Read the model definition and answer for the solid it produces. Units are mm, in the model's axes. A direction names the side the tool comes from. Coordinates: 2 decimals unless noted, no trailing zeros. Loops run counter-clockwise (first coordinate to the right, second up) from the corner with the lowest first, then second, coordinate; pieces in that order, holes last. Notation, with made-up numbers: (35, 85) -> (58, 85) arc R24 ccw to (58, 111) -> close; hole circle Ø5 at (67, 36). An arc over 180 degrees is marked (long way). Answer as a JSON object with one key per item and string values. Group by question number.
1) Determine the mould class of faces 1 (the face through (-17, 4, -63.5)), 2 (the face through (17, -1, -69.85)), 3 (the face through (-17, 4, 63.5)), 4 (the face through (1219.2, -40, 0)) for opening direction Z: released by +Z, released by -Z, zero draft, split by the parting line, or undercut.
2) Flat-ended cylindrical pins translate along their axes: P1, Ø1, axis at x = 168, z = -16.5, coming from the +Y side; P2, Ø15, axis at x = 291.29, z = 11.6, coming from the +Y side. Find the tip coordinate at first contact, or state that the pin passes through.
3) Section A-A, the plane y = -23 is taken. Give the vertices of the cut face in (x, z).
4) Consider probe 1 along Z at (x, y) = (596.5, 34); probe 2 along Y at (x, z) = (801, -51). Determine where each line is inside the solid, lowest interval first. Write a range as [from, to].
5) Section B-B, the plane x = 645 is taken. Give the vertices of the cut face in (y, z), plus the area to 3 significant figures.
6) Which of the six approach directions +Z, -Z, +X, -X, +Y, -Y give full straight-line access (tool end or side, diameter ignored) to faces 5 (the face through (-17, -38.1, -1)), 6 (the face through (17, -44.45, -1))?
from build123d import *

# Parameters (mm, degrees)
F0_W     = 88.9
F0_H     = 139.7
F1_DEPTH = 1219.2
F2_W     = 82.55
F2_H     = 127
F3_DEPTH = 2438.401
F4_R     = 12.7
F5_DEPTH = 88.901


with BuildPart() as f1:
    # F0 (on Right) → F1 (new body, symmetric)
    with BuildSketch(Plane.YZ):
        Rectangle(F0_W, F0_H)
    extrude(amount=F1_DEPTH, both=True)

    # F2 (on face) → F3 (cut, through all)
    with BuildSketch(Plane(origin=(-1219.2, 0, 0), x_dir=(0, -1, 0), z_dir=(-1, 0, 0))):
        with Locations((-3.175, 0)):
            Rectangle(F2_W, F2_H)
    extrude(amount=-F3_DEPTH, mode=Mode.SUBTRACT)

    # F4 (on face) → F5 (cut, through all)
    with BuildSketch(Plane.XZ.offset(44.45)):
        with BuildLine():
            ThreePointArc((-689.7858705791, 11.6012184261), (-694.2759986397, 9.7413464866), (-696.1358705791, 5.2512184261))
            Line((-696.1358705791, 5.2512184261), (-696.1358705791, -7.4487815739))
            ThreePointArc((-696.1358705791, -7.4487815739), (-694.2759986397, -11.9389096344), (-689.7858705791, -13.7987815739))
            ThreePointArc((-689.7858705791, -13.7987815739), (-685.2957425186, -11.9389096344), (-683.4358705791, -7.4487815739))
            Line((-683.4358705791, -7.4487815739), (-683.4358705791, 5.2512184261))
            ThreePointArc((-683.4358705791, 5.2512184261), (-685.2957425186, 9.7413464866), (-689.7858705791, 11.6012184261))
        make_face()
        with BuildLine():
            ThreePointArc((-537.3858705791, 14.7762184261), (-541.8759986397, 12.9163464866), (-543.7358705791, 8.4262184261))
            Line((-543.7358705791, 8.4262184261), (-543.7358705791, -4.2737815739))
            ThreePointArc((-543.7358705791, -4.2737815739), (-541.8759986397, -8.7639096344), (-537.3858705791, -10.6237815739))
            ThreePointArc((-537.3858705791, -10.6237815739), (-532.8957425186, -8.7639096344), (-531.0358705791, -4.2737815739))
            Line((-531.0358705791, -4.2737815739), (-531.0358705791, 8.4262184261))
            ThreePointArc((-531.0358705791, 8.4262184261), (-532.8957425186, 12.9163464866), (-537.3858705791, 14.7762184261))
        make_face()
        with BuildLine():
            ThreePointArc((-296.0858705791, 21.3802184261), (-300.5759986397, 19.5203464866), (-302.4358705791, 15.0302184261))
            Line((-302.4358705791, 15.0302184261), (-302.4358705791, 2.3302184261))
            ThreePointArc((-302.4358705791, 2.3302184261), (-300.5759986397, -2.1599096344), (-296.0858705791, -4.0197815739))
            ThreePointArc((-296.0858705791, -4.0197815739), (-291.5957425186, -2.1599096344), (-289.7358705791, 2.3302184261))
            Line((-289.7358705791, 2.3302184261), (-289.7358705791, 15.0302184261))
            ThreePointArc((-289.7358705791, 15.0302184261), (-291.5957425186, 19.5203464866), (-296.0858705791, 21.3802184261))
        make_face()
        with BuildLine():
            ThreePointArc((-242.1108705791, 21.3802184261), (-246.6009986397, 19.5203464866), (-248.4608705791, 15.0302184261))
            Line((-248.4608705791, 15.0302184261), (-248.4608705791, 2.3302184261))
            ThreePointArc((-248.4608705791, 2.3302184261), (-246.6009986397, -2.1599096344), (-242.1108705791, -4.0197815739))
            ThreePointArc((-242.1108705791, -4.0197815739), (-237.6207425186, -2.1599096344), (-235.7608705791, 2.3302184261))
            Line((-235.7608705791, 2.3302184261), (-235.7608705791, 15.0302184261))
            ThreePointArc((-235.7608705791, 15.0302184261), (-237.6207425186, 19.5203464866), (-242.1108705791, 21.3802184261))
        make_face()
        with BuildLine():
            ThreePointArc((-89.7108705791, 17.9512184261), (-94.2009986397, 16.0913464866), (-96.0608705791, 11.6012184261))
            Line((-96.0608705791, 11.6012184261), (-96.0608705791, -1.0987815739))
            ThreePointArc((-96.0608705791, -1.0987815739), (-94.2009986397, -5.5889096344), (-89.7108705791, -7.4487815739))
            ThreePointArc((-89.7108705791, -7.4487815739), (-85.2207425186, -5.5889096344), (-83.3608705791, -1.0987815739))
            Line((-83.3608705791, -1.0987815739), (-83.3608705791, 11.6012184261))
            ThreePointArc((-83.3608705791, 11.6012184261), (-85.2207425186, 16.0913464866), (-89.7108705791, 17.9512184261))
        make_face()
        with BuildLine():
            ThreePointArc((38.8766294209, 2.0762184261), (34.3865013603, 0.2163464866), (32.5266294209, -4.2737815739))
            Line((32.5266294209, -4.2737815739), (32.5266294209, -16.9737815739))
            ThreePointArc((32.5266294209, -16.9737815739), (34.3865013603, -21.4639096344), (38.8766294209, -23.3237815739))
            ThreePointArc((38.8766294209, -23.3237815739), (43.3667574814, -21.4639096344), (45.2266294209, -16.9737815739))
            Line((45.2266294209, -16.9737815739), (45.2266294209, -4.2737815739))
            ThreePointArc((45.2266294209, -4.2737815739), (43.3667574814, 0.2163464866), (38.8766294209, 2.0762184261))
        make_face()
        with BuildLine():
            ThreePointArc((69.0391294209, 17.9512184261), (64.5490013603, 16.0913464866), (62.6891294209, 11.6012184261))
            Line((62.6891294209, 11.6012184261), (62.6891294209, -1.0987815739))
            ThreePointArc((62.6891294209, -1.0987815739), (64.5490013603, -5.5889096344), (69.0391294209, -7.4487815739))
            ThreePointArc((69.0391294209, -7.4487815739), (73.5292574814, -5.5889096344), (75.3891294209, -1.0987815739))
            Line((75.3891294209, -1.0987815739), (75.3891294209, 11.6012184261))
            ThreePointArc((75.3891294209, 11.6012184261), (73.5292574814, 16.0913464866), (69.0391294209, 17.9512184261))
        make_face()
        with BuildLine():
            ThreePointArc((229.3766294209, 2.0762184261), (224.8865013603, 0.2163464866), (223.0266294209, -4.2737815739))
            Line((223.0266294209, -4.2737815739), (223.0266294209, -16.9737815739))
            ThreePointArc((223.0266294209, -16.9737815739), (224.8865013603, -21.4639096344), (229.3766294209, -23.3237815739))
            ThreePointArc((229.3766294209, -23.3237815739), (233.8667574814, -21.4639096344), (235.7266294209, -16.9737815739))
            Line((235.7266294209, -16.9737815739), (235.7266294209, -4.2737815739))
            ThreePointArc((235.7266294209, -4.2737815739), (233.8667574814, 0.2163464866), (229.3766294209, 2.0762184261))
        make_face()
        with BuildLine():
            ThreePointArc((386.5391294209, 22.7137184261), (382.0490013603, 20.8538464866), (380.1891294209, 16.3637184261))
            Line((380.1891294209, 16.3637184261), (380.1891294209, 3.6637184261))
            ThreePointArc((380.1891294209, 3.6637184261), (382.0490013603, -0.8264096344), (386.5391294209, -2.6862815739))
            ThreePointArc((386.5391294209, -2.6862815739), (391.0292574814, -0.8264096344), (392.8891294209, 3.6637184261))
            Line((392.8891294209, 3.6637184261), (392.8891294209, 16.3637184261))
            ThreePointArc((392.8891294209, 16.3637184261), (391.0292574814, 20.8538464866), (386.5391294209, 22.7137184261))
        make_face()
        with BuildLine():
            ThreePointArc((480.2016294209, 24.3012184261), (475.7115013603, 22.4413464866), (473.8516294209, 17.9512184261))
            Line((473.8516294209, 17.9512184261), (473.8516294209, 5.2512184261))
            ThreePointArc((473.8516294209, 5.2512184261), (475.7115013603, 0.7610903656), (480.2016294209, -1.0987815739))
            ThreePointArc((480.2016294209, -1.0987815739), (484.6917574814, 0.7610903656), (486.5516294209, 5.2512184261))
            Line((486.5516294209, 5.2512184261), (486.5516294209, 17.9512184261))
            ThreePointArc((486.5516294209, 17.9512184261), (484.6917574814, 22.4413464866), (480.2016294209, 24.3012184261))
        make_face()
        with BuildLine():
            ThreePointArc((605.6141294209, 5.5687184261), (601.1240013603, 3.7088464866), (599.2641294209, -0.7812815739))
            Line((599.2641294209, -0.7812815739), (599.2641294209, -16.6562815739))
            ThreePointArc((599.2641294209, -16.6562815739), (601.1240013603, -21.1464096344), (605.6141294209, -23.0062815739))
            ThreePointArc((605.6141294209, -23.0062815739), (610.1042574814, -21.1464096344), (611.9641294209, -16.6562815739))
            Line((611.9641294209, -16.6562815739), (611.9641294209, -0.7812815739))
            ThreePointArc((611.9641294209, -0.7812815739), (610.1042574814, 3.7088464866), (605.6141294209, 5.5687184261))
        make_face()
        with Locations((167.4641294209, 11.6012184261)):
            Circle(F4_R)
        with Locations((291.2891294209, 11.6012184261)):
            Circle(F4_R)
        with Locations((291.2891294209, -39.1987815739)):
            Circle(F4_R)
        with Locations((167.4641294209, -39.1987815739)):
            Circle(F4_R)
    extrude(amount=-F5_DEPTH, mode=Mode.SUBTRACT)


solid = f1.part
Determined:
{
 "1": {"face 1": "undercut", "face 2": "released by -Z", "face 3": "undercut", "face 4": "zero draft"},
 "2": {"P1": "y = -38.1", "P2": "through"},
 "3": {"outline": "(-1219.2, -69.85) -> (1219.2, -69.85) -> (1219.2, -63.5) -> (-1219.2, -63.5) -> close; (-1219.2, 63.5) -> (1219.2, 63.5) -> (1219.2, 69.85) -> (-1219.2, 69.85) -> close"},
 "4": {"probe 1": "[-69.85, -63.5], [63.5, 69.85]", "probe 2": "[-44.45, -38.1]"},
 "5": {"outline": "(-44.45, -69.85) -> (44.45, -69.85) -> (44.45, -63.5) -> (-38.1, -63.5) -> (-38.1, 63.5) -> (44.45, 63.5) -> (44.45, 69.85) -> (-44.45, 69.85) -> close", "area": "1,940 mm²"},
 "6": {"face 5": "+X, -X, +Y", "face 6": "+Z, -Z, +X, -X, -Y"}
}
